Source: three-view drawing plus pictorial views. Frame: mm from the lowest corner of the part. A direction names the side the tool comes from. Give positions to 0.01 mm unless a question says otherwise; leave off trailing zeros. Order: outer loops, then holes, each group sorted by start corner. A loop starts at its lowest first (then second) coordinate and runs counter-clockwise, first axis right, second up.
1) Access query for the marked faces 1, 2 and 3. Directions: +Z, -Z, +X, -X, +Y, -Y. A direction counts if a zero-diameter tool reaches every point of the face in a straight line with its end or side. Return the directions, or none.
2) Section C-C, the plane z = 13.25. Return loops of the section in (x, y), plus the area to 3 significant figures.
3) Section D-D, the plane y = 32. Return loops of the section in (x, z).
4) Section A-A, the plane x = 51.05. Return loops of the section in (y, z).
5) Section B-B, the plane z = 7.5. Return loops of the section in (x, y).
6) First-contact query: P1, Ø7.5, axis at x = 55, z = 8.5, coming from the +Y side; P2, Ø1.5, axis at y = 5.5, z = 11, coming from the -X side; P3, Ø4, axis at x = 31, z = 12, coming from the -Y side. Flat tips, straight axial feed; report the tip coordinate or a pass-through.
7) Material intervals for line 1 (Z direction, x = 51.05, y = 2); line 2 (X direction, y = 2.15, z = 7.5); line 3 (X direction, y = 11.5, z = 9.5), sorted ascending.
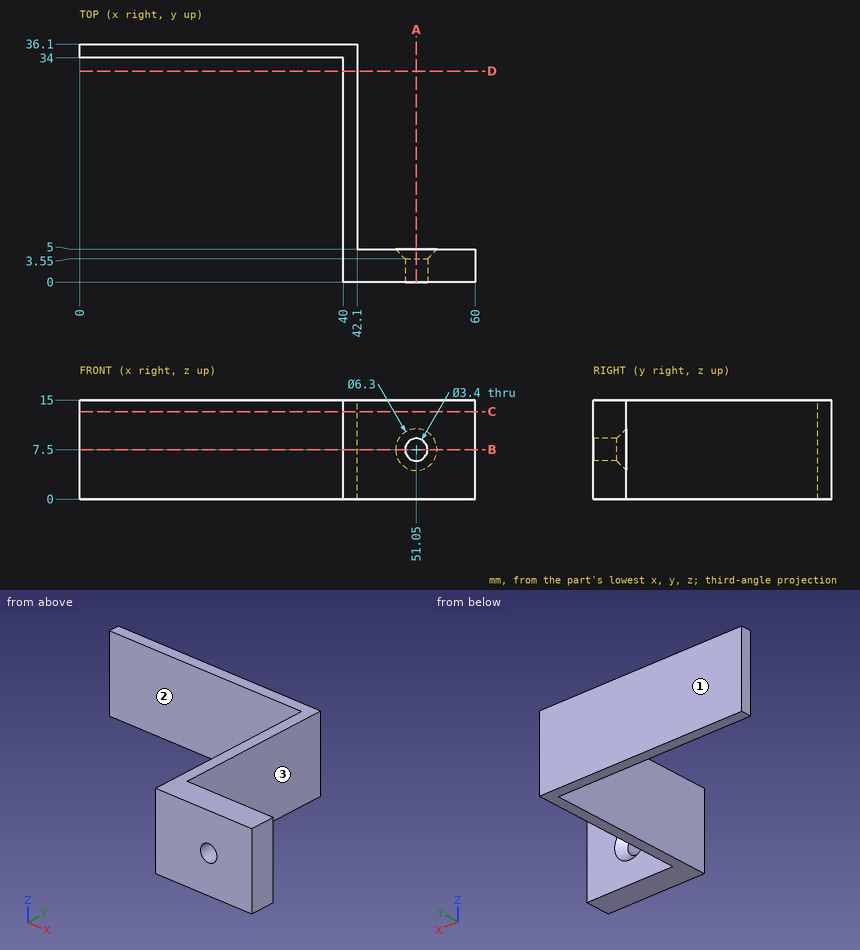
From the geometry:
1. face 1: +Z, -Z, +X, -X, +Y
1. face 2: +Z, -Z, -X, -Y
1. face 3: +Z, -Z, +X, +Y
2. outline: (0, 34) - (40, 34) - (40, 0) - (60, 0) - (60, 5) - (42.1, 5) - (42.1, 36.1) - (0, 36.1) - close
2. area: 249 mm2
3. outline: (40, 0) - (42.1, 0) - (42.1, 15) - (40, 15) - close
4. outline: (0, 0) - (5, 0) - (5, 4.35) - (3.55, 5.8) - (0, 5.8) - close; (0, 9.2) - (3.55, 9.2) - (5, 10.65) - (5, 15) - (0, 15) - close
5. outline: (0, 34) - (40, 34) - (40, 0) - (49.35, 0) - (49.35, 3.55) - (47.9, 5) - (42.1, 5) - (42.1, 36.1) - (0, 36.1) - close; (52.75, 0) - (60, 0) - (60, 5) - (54.2, 5) - (52.75, 3.55) - close
6. P1: stops at y = 5
6. P2: stops at x = 40
6. P3: stops at y = 34
7. line 1: z = 0 to 5.8, 9.2 to 15
7. line 2: x = 40 to 49.35, 52.75 to 60
7. line 3: x = 40 to 42.1
